Answer from the drawing. Dimensions are ordinates in mm from the lowest x, y and z of the part. A direction names the side the tool comes from. Round coordinates to 2 decimals unless told otherwise and drop trailing zeros. Loops run counter-clockwise (first coordinate to the right, second up) from the corner with the lowest first, then second, coordinate; pieces in that order, holes last. Notation, with made-up numbers: M 84,-36.5 L 131,-36.5 A20 ccw 131,-19.5 Z; hole C -1,-37 d5. An arc over 180 degrees is marked long. Write each question's results on one line, items separated by ' | '.
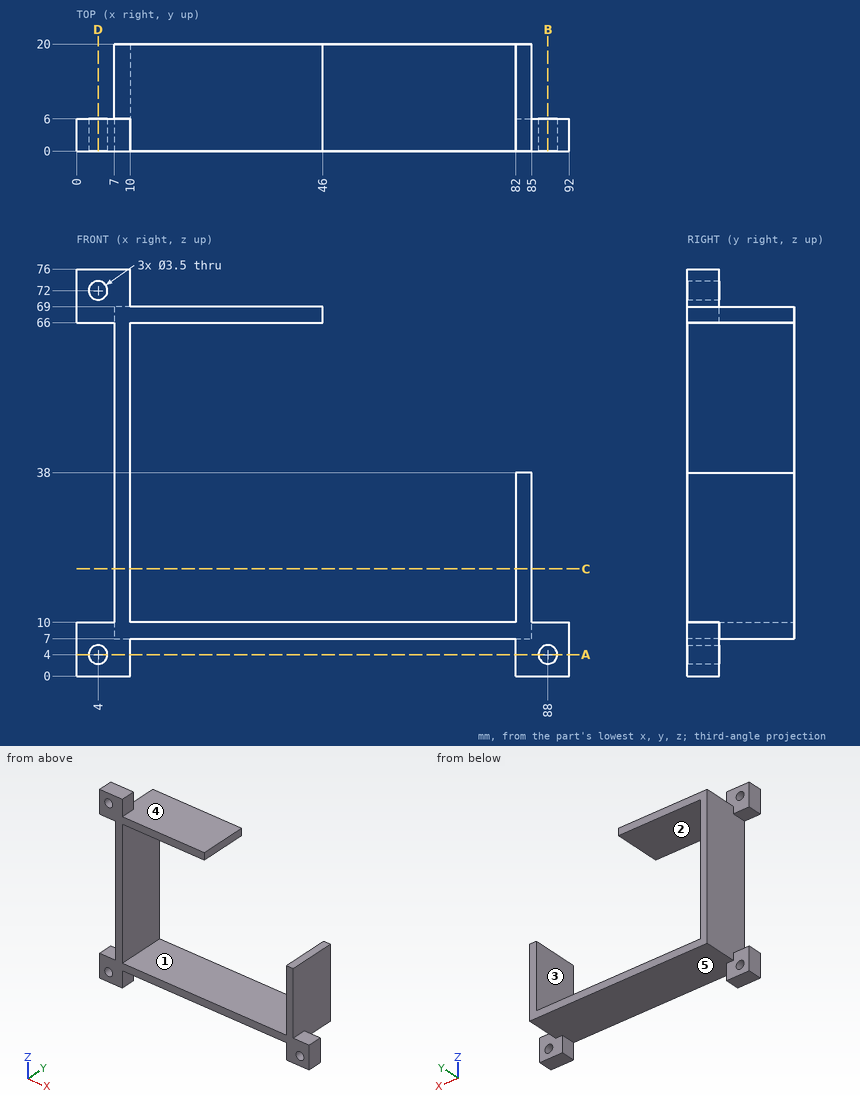
1. Find section C-C, the plane z = 20. Give the vertices of the cut face in (x, y).
Completed:
outline: M 7,0 L 10,0 L 10,20 L 7,20 Z; M 82,0 L 85,0 L 85,20 L 82,20 Z
2. Given P1, Ø5, axis at x = 15.5, y = 4, coming from the -Z side; P2, Ø2, axis at x = 88, z = 4, coming from the +Y side (3 decimals); P3, Ø1.5, axis at x = 84, y = 13.5, coming from the +Z side; P4, Ø2.5, axis at y = 13, z = 67.5, coming from the +X side, each flat-ended and moving along its own axis, determine where each tip first touches the part or whether it passes through.
Completed:
P1: stops at z = 7 | P2: passes through | P3: stops at z = 38 | P4: stops at x = 46
3. Find section A-A, the plane z = 4. Give the vertices of the cut face in (x, y), then the cut area to 3 significant figures.
Completed:
outline: M 0,0 L 2.25,0 L 2.25,6 L 0,6 Z; M 5.75,0 L 10,0 L 10,6 L 5.75,6 Z; M 82,0 L 86.25,0 L 86.25,6 L 82,6 Z; M 89.75,0 L 92,0 L 92,6 L 89.75,6 Z | area: 78.0 mm2
4. Find the intervals of material crossed by L1, parallel to X at y = 2.15, z = 4; L2, parallel to X at y = 1.75, z = 72; L3, parallel to X at y = 10, z = 32, in increasing order.
Completed:
L1: x = 0 to 2.25, 5.75 to 10, 82 to 86.25, 89.75 to 92 | L2: x = 0 to 2.25, 5.75 to 10 | L3: x = 7 to 10, 82 to 85
5. Which of the six approach directions +Z, -Z, +X, -X, +Y, -Y give full straight-line access (tool end or side, diameter ignored) to the marked faces 1 and 2?
Completed:
face 1: +Y, -Y | face 2: +X, +Y, -Y
6. Find section D-D, the plane x = 4. Give the vertices of the cut face in (y, z).
Completed:
outline: M 0,0 L 6,0 L 6,2.25 L 0,2.25 Z; M 0,5.75 L 6,5.75 L 6,10 L 0,10 Z; M 0,66 L 6,66 L 6,70.25 L 0,70.25 Z; M 0,73.75 L 6,73.75 L 6,76 L 0,76 Z
7. Determine the mould class of the marked faces 3, 4 and 5 for opening direction X: released by +X, released by -X, zero draft, split by the parting line, or undercut.
Completed:
face 3: undercut | face 4: zero draft | face 5: undercut
8. Find section B-B, the plane x = 88. Give the vertices of the cut face in (y, z).
Completed:
outline: M 0,0 L 6,0 L 6,2.25 L 0,2.25 Z; M 0,5.75 L 6,5.75 L 6,10 L 0,10 Z
